```python
from build123d import *

# Parameters (mm, degrees)
SKETCH_1_R          = 2.07
SKETCH_1_R_2        = 4.25
EXTRUDE_1_DEPTH     = 7
SKETCH_2_R          = 6.5
CUT_EXTRUDE_1_DEPTH = 5
SKETCH_3_R          = 2.07
CUT_EXTRUDE_2_DEPTH = 72.639587412


with BuildPart() as part:
    # 草图1 → 凸台-拉伸1 (new body)
    with BuildSketch(Plane.XY):
        with BuildLine():
            ThreePointArc((13.001837611, 43.091271905), (12.051039078, 35.055565267), (8.987193751, 27.566276194))
            Line((8.987193751, 27.566276194), (4.614556012, 19.992645468))
            ThreePointArc((4.614556012, 19.992645468), (0.106016193, 14.041662919), (-5.732396759, 9.388270735))
            ThreePointArc((-5.732396759, 9.388270735), (-10.589404565, -2.977332859), (0, -11))
            Line((0, -11), (35, -11))
            ThreePointArc((35, -11), (42.071067812, -8.071067812), (45, -1))
            Line((45, -1), (45, 29.980762114))
            ThreePointArc((45, 29.980762114), (44.659258263, 32.568952565), (43.660254038, 34.980762114))
            Line((43.660254038, 34.980762114), (35.392304845, 49.301270189))
            ThreePointArc((35.392304845, 49.301270189), (31, 53.693575035), (25, 55.301270189))
            ThreePointArc((25, 55.301270189), (16.440795031, 51.711978263), (13.001837611, 43.091271905))
        make_face()
        Circle(SKETCH_1_R, mode=Mode.SUBTRACT)
        with Locations((35, 1)):
            Circle(SKETCH_1_R, mode=Mode.SUBTRACT)
        with Locations((35, 16)):
            Circle(SKETCH_1_R, mode=Mode.SUBTRACT)
        with Locations((25, 43.301270189)):
            Circle(SKETCH_1_R_2, mode=Mode.SUBTRACT)
    extrude(amount=EXTRUDE_1_DEPTH)

    # 草图2 → 切除-拉伸1 (cut)
    with BuildSketch(Plane.XY.offset(7)):
        with Locations((25, 43.301270189)):
            Circle(SKETCH_2_R)
    extrude(amount=-CUT_EXTRUDE_1_DEPTH, mode=Mode.SUBTRACT)

    # 草图3 → 切除-拉伸2 (cut, through all)
    with BuildSketch(Plane.XY.offset(7)):
        with Locations((20, 0)):
            Circle(SKETCH_3_R)
    extrude(amount=-CUT_EXTRUDE_2_DEPTH, mode=Mode.SUBTRACT)


solid = part.part
```
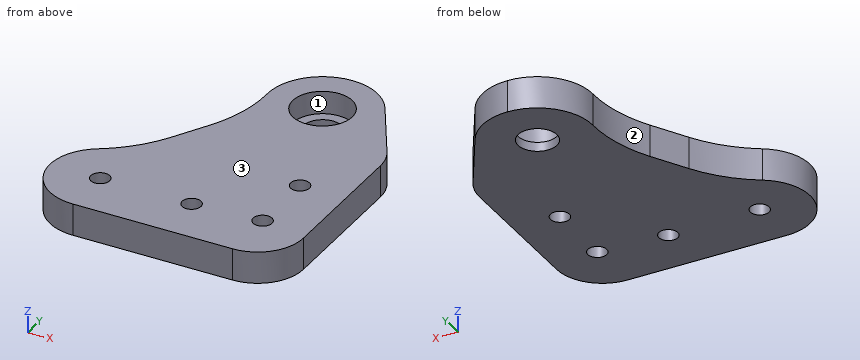
Verification items for the finished model (mm, model axes). Face numbers are marked on the shaded views. Round coordinates to 2 decimals unless told otherwise and drop trailing zeros. Order: outer loops, then holes, each group sorted by start corner. A loop starts at its lowest first (then second) coordinate and runs counter-clockwise, first axis right, second up. Notation, with made-up numbers: (33, 83) - (62, 83) arc R19 ccw to (62, 116) - close; hole circle Ø6 at (-36.5, -5). An arc over 180 degrees is marked (long way). Use CSV: the item, a comma, the result in double quotes. Start each with the question number.
1) Mould release check, pull along X, two halves, no side actions. Record for the marked faces 1, 2 and 3: +X half, -X half, draft (parallel to the pull), parting line (faces both ways), or undercut.
2) Section check B-B, the plane y = 15. Record the cut outline in (x, z).
3) Section check A-A, the plane x = 1. Record the cut outline in (y, z), plus the area to 3 significant figures.
4) Thickness scan on L1, parallel to Y at x = 25, z = 0.75; L2, parallel to Y at x = 20, z = 3.5; L3, parallel to Y at x = 35.5, z = 4. Record the ranges inside material, lowest first.
5) Section check D-D, the plane x = 20. Record the cut outline in (y, z).
6) Go/stop test with flat-tipped pins: P1, Ø6.5, axis at x = 24.5, y = 41.5, coming from the +Z side; P2, Ø4, axis at x = 39, z = 1, coming from the +Y side; P3, Ø3, axis at y = 22.5, z = 5, coming from the -X side; P4, Ø3.5, axis at x = 35, y = 1, coming from the -Z side. Record where each tip stops, or that it passes through.
7) Section check C-C, the plane z = 6. Record the cut outline in (x, y).
Answers:
1,face 1,"undercut"
1,face 2,"-X half"
1,face 3,"draft"
2,outline,"(1, 0) - (33.19, 0) - (33.19, 7) - (1, 7) - close; (36.81, 0) - (45, 0) - (45, 7) - (36.81, 7) - close"
3,outline,"(-11, 0) - (-1.81, 0) - (-1.81, 7) - (-11, 7) - close; (1.81, 0) - (15, 0) - (15, 7) - (1.81, 7) - close"
3,area,"157 mm²"
4,L1,"y = -11 to 39.05, 47.55 to 55.3"
4,L2,"y = -11 to -2.07, 2.07 to 39.15, 47.45 to 54.21"
4,L3,"y = -10.99 to -1.01, 3.01 to 13.99, 18.01 to 49.11"
5,outline,"(-11, 0) - (-2.07, 0) - (-2.07, 7) - (-11, 7) - close; (2.07, 0) - (54.21, 0) - (54.21, 7) - (47.45, 7) - (47.45, 2) - (39.15, 2) - (39.15, 7) - (2.07, 7) - close"
6,P1,"stops at z = 2"
6,P2,"stops at y = 46.52"
6,P3,"stops at x = 5.2"
6,P4,"passes through"
7,outline,"(-5.73, 9.39) arc R11 ccw to (0, -11) - (35, -11) arc R10 ccw to (45, -1) - (45, 29.98) arc R10 ccw to (43.66, 34.98) - (35.39, 49.3) arc R12 ccw to (13, 43.09) arc R30 cw to (8.99, 27.57) - (4.61, 19.99) arc R30 cw to start; hole circle Ø4.14 at (0, 0); hole circle Ø4.14 at (20, 0); hole circle Ø13 at (25, 43.3); hole circle Ø4.14 at (35, 1); hole circle Ø4.14 at (35, 16)"
